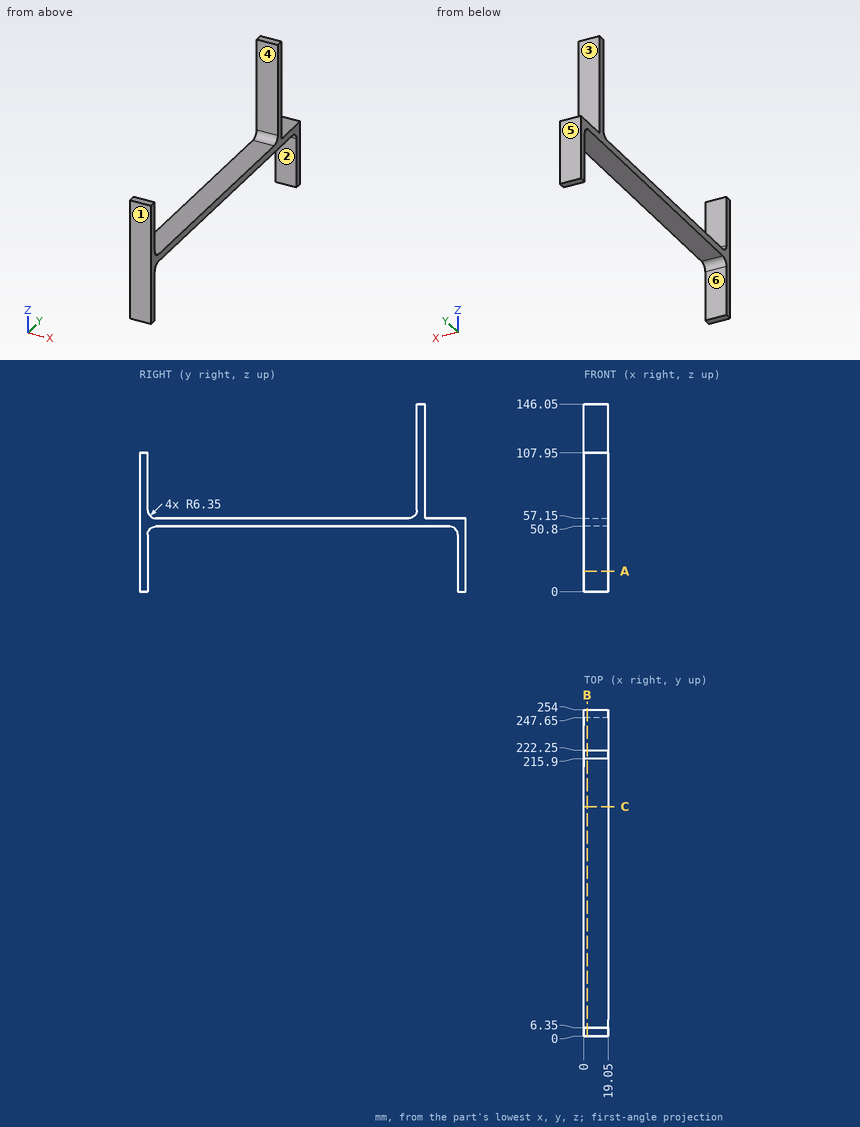
Check sheet for the drawn part. Datum: minimum x, y, z corner. Units: mm. A direction names the side the tool comes from. Give positions to 0.01 mm unless a question says otherwise; leave off trailing zeros. Order: outer loops, then holes, each group sorted by start corner. A loop starts at its lowest first (then second) coordinate and runs counter-clockwise, first axis right, second up.
1. Sectioned sample at B-B (x = 2.5). Record the boundary of the cut face in (y, z), then the cut area to 3 significant figures.
Completed:
outline: (0, 0) - (6.35, 0) - (6.35, 44.45) arc R6.35 cw to (12.7, 50.8) - (241.3, 50.8) arc R6.35 cw to (247.65, 44.45) - (247.65, 0) - (254, 0) - (254, 57.15) - (222.25, 57.15) - (222.25, 146.05) - (215.9, 146.05) - (215.9, 63.5) arc R6.35 cw to (209.55, 57.15) - (12.7, 57.15) arc R6.35 cw to (6.35, 63.5) - (6.35, 107.95) - (0, 107.95) - close
area: 3,180 mm2
2. Sectioned sample at A-A (z = 16). Record the boundary of the cut face in (x, y), then the cut area to 3 significant figures.
Completed:
outline: (0, 0) - (19.05, 0) - (19.05, 6.35) - (0, 6.35) - close; (0, 247.65) - (19.05, 247.65) - (19.05, 254) - (0, 254) - close
area: 242 mm2
3. Depth check by flat-ended pin: pin 1 (9.5 mm diameter, centred on x = 5.5, y = 71.5, fed in from +Z); pin 2 (6 mm diameter, centred on x = 17, z = 70, fed in from +Y); pin 3 (9.5 mm diameter, centred on x = 6, z = 97, fed in from -Y); pin 4 (1 mm diameter, centred on x = 15, y = 187.5, fed in from -Z). Enter the tip coordinate at first touch or a pass-through.
Completed:
pin 1: stops at z = 57.15
pin 2: stops at y = 222.25
pin 3: stops at y = 0
pin 4: stops at z = 50.8
4. Scan lines: line 1 (Y direction, x = 14.25, z = 32.5); line 2 (Y direction, x = 7.75, z = 103); line 3 (Z direction, x = 10.75, y = 98). Record each from-to range of solid material in increasing order.
Completed:
line 1: y = 0 to 6.35, 247.65 to 254
line 2: y = 0 to 6.35, 215.9 to 222.25
line 3: z = 50.8 to 57.15
5. Draft check along Y on the marked faces 1, 2 and 3. Enter one of: pulls with the +Y half, pulls with the -Y half, needs draft (parallel to the pull), parting line crosses it, or undercut.
Completed:
face 1: pulls with the -Y half
face 2: undercut
face 3: pulls with the +Y half
6. Access from +Z, -Z, +X, -X, +Y, -Y to the whole of each face (thin tool, end or side, straight path). Record for the marked faces 4, 5 and 6.
Completed:
face 4: +Z, +X, -X
face 5: +Z, -Z, +X, -X, +Y
face 6: -Z, +X, -X
7. Sectioned sample at C-C (y = 178.5). Record the boundary of the cut face in (x, z).
Completed:
outline: (0, 50.8) - (19.05, 50.8) - (19.05, 57.15) - (0, 57.15) - close
